Input: dimensioned drawing with shaded views. Units: mm. Origin: part minimum x, y, z. A direction names the side the tool comes from. Coordinates: 2 decimals unless noted, no trailing zeros. Write each loop counter-clockwise with the first axis right and the second up, starting at its lowest first coordinate (ties: lowest second). Pieces come first, ordered by that corner, then holes. Notation, with made-up numbers: (-33, -23) -> (-28, -23) arc R32 ccw to (-28, 16) -> close; hole circle Ø1 at (-8, 63). An arc over 180 degrees is marked (long way). One line per item, written item: value. Start each with the question number.
1. Mould query, pull axis Y, two halves, no side actions, for the marked faces 1, 2 and 3. Classes: released by +Y, released by -Y, zero draft, split by the parting line, or undercut.
2. Section query C-C, the plane z = 39. Output: boundary loops of the cut face in (x, y) (3 decimals), and give its area (3 significant figures).
3. Line query: line 1 (Y direction, x = 150, z = 5); line 2 (Z direction, x = 199.5, y = 353); line 3 (X direction, y = 267, z = 72.5). Output: solid intervals per line, ascending.
4. Section query A-A, the plane y = 270. Output: boundary loops of the cut face in (x, z), and give its area (3 significant figures).
5. Access query for the marked faces 4, 5 and 6. Directions: +Z, -Z, +X, -X, +Y, -Y. A direction counts if a zero-diameter tool reaches every point of the face in a straight line with its end or side. Return the directions, or none.
6. Section query B-B, the plane x = 163. Output: boundary loops of the cut face in (y, z), and give its area (3 significant figures).
7. Section query D-D, the plane y = 65.5. Output: boundary loops of the cut face in (x, z), and give its area (3 significant figures).
8. First-contact query: P1, Ø8, axis at x = 263, z = 40.5, coming from the +Y side; P2, Ø6, axis at y = 319, z = 66, coming from the +X side; P3, Ø12, axis at y = 299, z = 35, coming from the +X side. Flat tips, straight axial feed; report the tip coordinate or a pass-through.
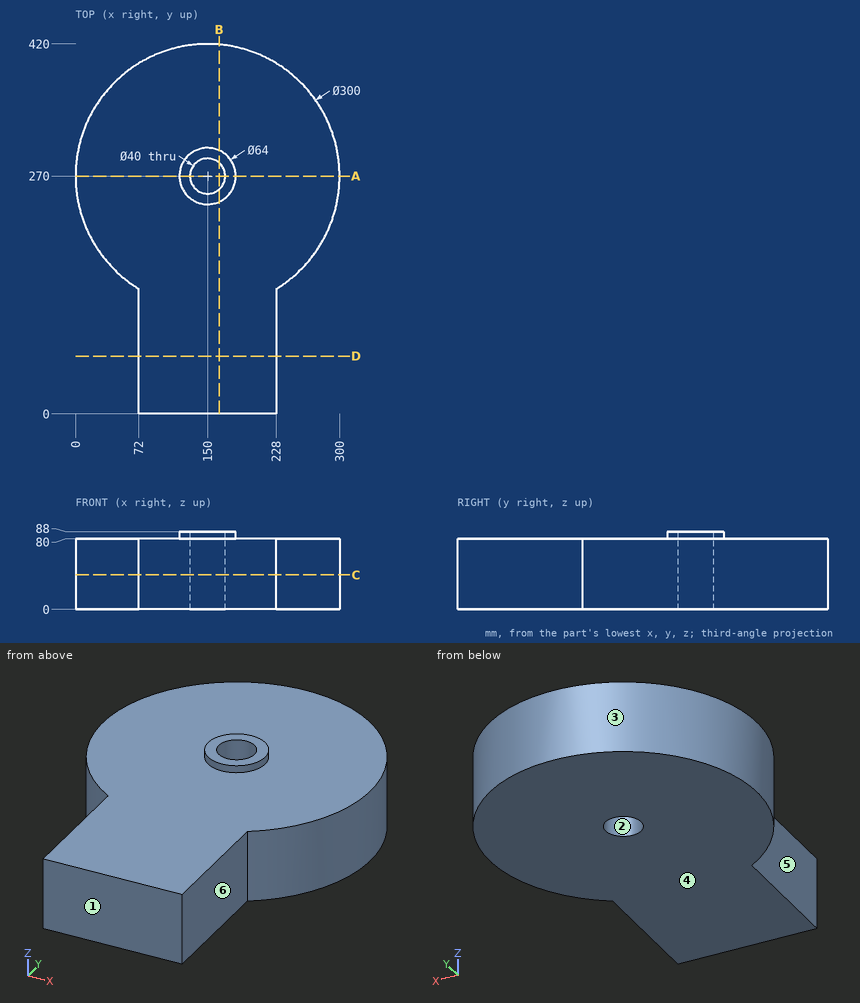
Computed values:
1. face 1: released by -Y
1. face 2: undercut
1. face 3: split by the parting line
2. outline: (72, 0) -> (228, 0) -> (228, 141.875) arc R150 ccw (long way) to (72, 141.875) -> close; hole circle Ø40 at (150, 270)
2. area: 89,300 mm²
3. line 1: y = 0 to 250, 290 to 420
3. line 2: z = 0 to 80
3. line 3: x = 0.03 to 130.23, 169.77 to 299.97
4. outline: (0, 0) -> (130, 0) -> (130, 88) -> (118, 88) -> (118, 80) -> (0, 80) -> close; (170, 0) -> (300, 0) -> (300, 80) -> (182, 80) -> (182, 88) -> (170, 88) -> close
4. area: 21,000 mm²
5. face 4: -Z, +X, -X, +Y, -Y
5. face 5: +Z, -Z, -X, -Y
5. face 6: +Z, -Z, +X, -Y
6. outline: (0, 0) -> (254.8, 0) -> (254.8, 88) -> (240.76, 88) -> (240.76, 80) -> (0, 80) -> close; (285.2, 0) -> (419.44, 0) -> (419.44, 80) -> (299.24, 80) -> (299.24, 88) -> (285.2, 88) -> close
6. area: 31,300 mm²
7. outline: (72, 0) -> (228, 0) -> (228, 80) -> (72, 80) -> close
7. area: 12,500 mm²
8. P1: stops at y = 373.05
8. P2: stops at x = 292.77
8. P3: stops at x = 298.23
